The figure shows three views and two pictorial views of one solid part (mm, origin at its lowest corner). Answer the questions. Coordinates: 2 decimals unless noted, no trailing zeros. Loops run counter-clockwise (first coordinate to the right, second up) from the corner with the lowest first, then second, coordinate; pieces in that order, holes last. Notation, with made-up numbers: M -5,21.5 L 15,21.5 A13 cw 15,44.5 Z; hole C -29.75,80.25 d1. An arc over 180 degrees is marked long. Answer as a JSON object with one key per item and string values. Group by question number.
1. A cutting plane is placed at C-C on x = 5.75. Give the vertices of the cut face in (y, z).
2. Straight lines are drawn through the part: L1, parallel to X at y = 1.6, z = 50.5; L2, parallel to Z at x = 16.75, y = 1.1; L3, parallel to Z at x = 21.5, y = 1.4. For each, find the intervals that lie inside material, in ascending order.
3. A cutting plane is placed at A-A on z = 52.5. Give the vertices of the cut face in (x, y).
4. A cutting plane is placed at B-B on y = 0.4. Give the vertices of the cut face in (x, z).
5. Given pin 1 (6 mm diameter, centred on x = 15, z = 37, fed in from -Y), flat-ended and moving along its own axis, determine where the tip first touches the part or whether it passes through.
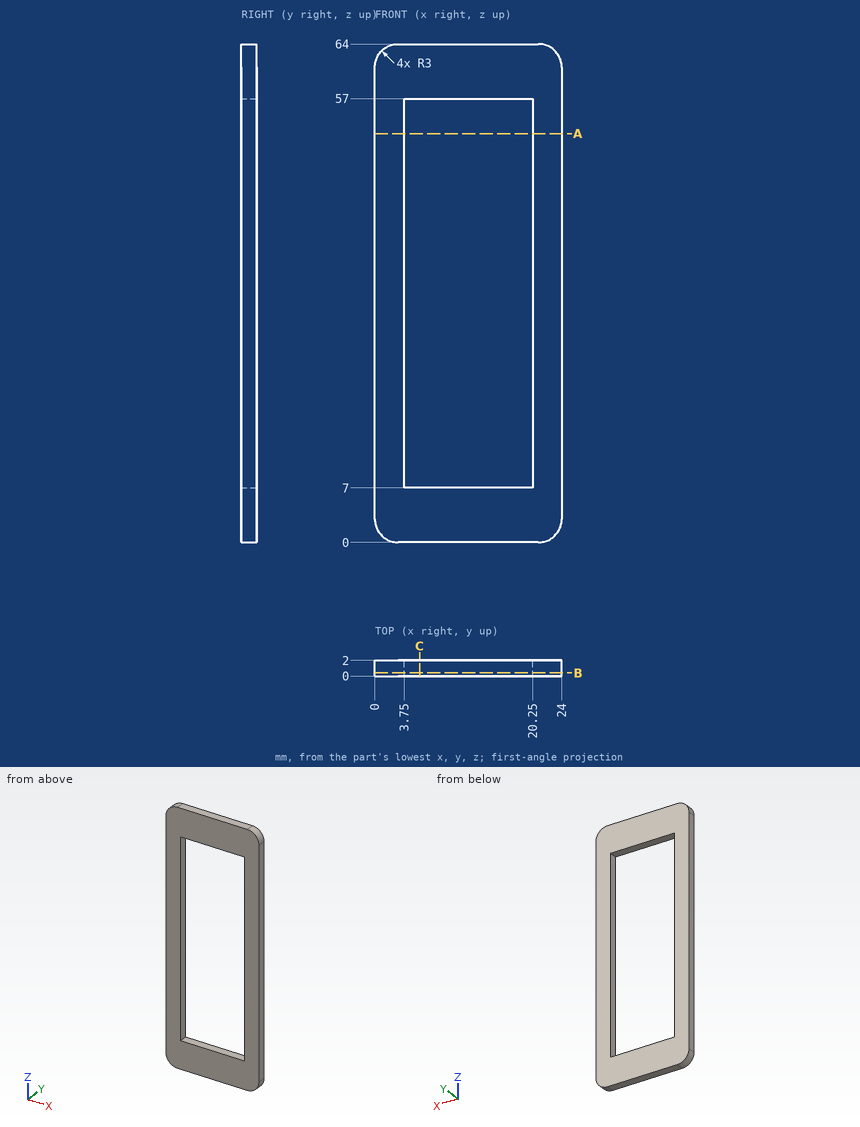
From the geometry:
{
 "1": {"outline": "M 0,0 L 2,0 L 2,7 L 0,7 Z; M 0,57 L 2,57 L 2,64 L 0,64 Z"},
 "2": {"L1": "x = 0 to 3.75, 20.25 to 24", "L2": "z = 0 to 7, 57 to 64", "L3": "z = 0.04 to 63.96"},
 "3": {"outline": "M 0,0 L 3.75,0 L 3.75,2 L 0,2 Z; M 20.25,0 L 24,0 L 24,2 L 20.25,2 Z"},
 "4": {"outline": "M 0,3 A3 ccw 3,0 L 21,0 A3 ccw 24,3 L 24,61 A3 ccw 21,64 L 3,64 A3 ccw 0,61 Z; hole M 3.75,7 L 20.25,7 L 20.25,57 L 3.75,57 Z"},
 "5": {"pin 1": "passes through"}
}
